The listing builds one solid part. Answer for the finished solid, in the listing's coordinates (mm). A direction names the side the tool comes from. Coordinates: 2 decimals unless noted, no trailing zeros. Write each loop counter-clockwise with the first axis right and the second up, starting at its lowest first coordinate (ties: lowest second). Pieces come first, ordered by that corner, then holes. Notation, with made-up numbers: M 22,-19 L 53,-19 A14 cw 53,0 Z; hole C -22,-22.75 d2. An arc over 180 degrees is marked long. Answer as a JSON object with one key per item and string values. Group by question number.
from build123d import *

# Parameters (mm, degrees)
BASE_FLANGE1_DEPTH = 114.3
SKETCH6_W          = 50.8
SKETCH6_H          = 733.425
TAB1_DEPTH         = 3.175


# Sheet-metal steps are written as plain solids
with BuildPart() as part:
    # Sketch1 → Base-Flange1 (new, symmetric)
    with BuildSketch(Plane(origin=(0, 0, 0), x_dir=(0, 0, -1), z_dir=(1, 0, 0))):
        with BuildLine():
            Line((-95.25, 0), (-0.7366, 0))
            ThreePointArc((-0.7366, 0), (-0.215745145, 0.215745145), (0, 0.7366))
            Line((0, 0.7366), (0, 762))
            Line((0, 762), (3.175, 762))
            Line((3.175, 762), (3.175, 0.7366))
            ThreePointArc((3.175, 0.7366), (2.029318885, -2.029318885), (-0.7366, -3.175))
            Line((-0.7366, -3.175), (-95.25, -3.175))
            Line((-95.25, -3.175), (-95.25, 0))
        make_face()
    extrude(amount=BASE_FLANGE1_DEPTH, both=True)

    # Sketch6 → Tab1 (add)
    with BuildSketch(Plane(origin=(0, 0, -3.175), x_dir=(-1, 0, 0), z_dir=(0, 0, -1))):
        with Locations((-139.7, 395.2875)):
            Rectangle(SKETCH6_W, SKETCH6_H)
        with Locations((139.7, 395.2875)):
            Rectangle(SKETCH6_W, SKETCH6_H)
    extrude(amount=-TAB1_DEPTH)


solid = part.part
Item 1: A cutting plane is placed at A-A, the plane x = -44. Write down the section's boundary in (y, z) (3 decimals).
Item 2: A cutting plane is placed at C-C, the plane z = 53. Write down the section's boundary in (x, y) (3 decimals).
Item 3: Consider L1, parallel to Y at x = 67.5, z = 52 (3 decimals). Determine where the line is inside the solid, lowest interval first. Write a range as from..to.
Item 4: A cutting plane is placed at B-B, the plane y = 540. Write down the section's boundary in (x, z) (3 decimals).
Item 5: Flat-ended cylindrical pins translate along their axes: pin 1 Ø5 at (x, y) = (-119.5, 325.5) entering from +Z; pin 2 Ø16 at (y, z) = (14, 36.5) entering from -X; pin 3 Ø6 at (x, z) = (17.5, 79) entering from +Y; pin 4 Ø3.5 at (x, z) = (-134, -1) entering from -Y (3 decimals). Find the tip coordinate at first contact, or state that the pin passes through.
Item 6: A tool of negligible diameter and unlimited length cuts with its end or side. For faces 1 (the face through (-114.3, -0.2, 34.9)), 2 (the face through (114.3, -0.2, 34.9)), 3 (the face through (2, 387, -3.175)), 4 (the face through (2, 0, 49)), from which of +Z, -Z, +X, -X, +Y, -Y can it reach the whole face along a straight path? Write none if from no direction.
Answer:
{
 "1": {"outline": "M -3.175,0.737 A3.912 ccw 0.737,-3.175 L 762,-3.175 L 762,0 L 0.737,0 A0.737 cw 0,0.737 L 0,95.25 L -3.175,95.25 Z"},
 "2": {"outline": "M -114.3,-3.175 L 114.3,-3.175 L 114.3,0 L -114.3,0 Z"},
 "3": {"L1": "-3.175..0"},
 "4": {"outline": "M -165.1,-3.175 L 165.1,-3.175 L 165.1,0 L -165.1,0 Z"},
 "5": {"pin 1": "z = 0", "pin 2": "through", "pin 3": "y = 0", "pin 4": "y = 28.575"},
 "6": {"face 1": "+Z, -Z, -X, -Y", "face 2": "+Z, -Z, +X, -Y", "face 3": "-Z, +X, -X, +Y, -Y", "face 4": "+Z, +X, -X, +Y"}
}
